The model under review builds one solid part; all positions refer to its coordinate system, in mm. A direction names the side the tool comes from. Round coordinates to 2 decimals unless told otherwise and drop trailing zeros. Loops run counter-clockwise (first coordinate to the right, second up) from the corner with the lowest first, then second, coordinate; pieces in that order, holes last. Notation, with made-up numbers: M 8.25,16.25 L 67.25,16.25 A14 cw 67.25,21.25 Z; hole C 67,62.5 d1. An arc over 180 degrees is marked long. Return JSON: item names as keys, results as strings. Group by question number.
Q1. To check wall thickness, follow line 1 along X through (y, z) = (16.3, 0); line 2 along Y through (x, z) = (17.5, 47); line 3 along Y through (x, z) = (25, 32.25). State the ranges of each line that lie inside material, in increasing order.
Q2. Consider section C-C (y = -46). State the section outline as (x, z) points.
Q3. Consider section B-B (z = -33). Count the separate pieces of the cut face and the enclosed holes in it, and give its area (3 significant figures).
Q4. Draft analysis for pull direction Y (two halves, no side actions). For faces 1 (the face through (15.69, -17.46, -49.84)), 2 (the face through (-34, -86.15, -14)), 3 (the face through (27.147, 68.608, 32.475)), state which applies: pulls with the +Y half, pulls with the -Y half, needs draft (parallel to the pull), parting line crosses it, or undercut.
Q5. Clearance check with flat-ended pins moving along their axes: pin 1 Ø5.5 at (x, y) = (25, 86.5) entering from -Z; pin 2 Ø4 at (x, y) = (25, 68.5) entering from +Z; pin 3 Ø1 at (x, y) = (1.5, 49.5) entering from +Z; pin 4 Ø5 at (x, y) = (5.5, 30) entering from +Z. State where each tip first meets the part, or that it passes through.
Q6. Consider section A-A (y = 68.5). State the section outline as (x, z) points, and give its area (3 significant figures).
Q7. For faces 4 (the face through (29.23, -0.21, -31.88)), 5 (the face through (-35, -92.5, 16)), 6 (the face through (-34, 13.85, -14)), 7 (the face through (-23, -62.5, 37)), list the 3-axis set-ups (+Z, -Z, +X, -X, +Y, -Y) from which the entire face can be reached by the end or side of a thin tool; tool diameter is ignored.
from build123d import *

# Parameters (mm, degrees)
SKETCH1_R                      = 45.25
SKETCH1_R_2                    = 38.25
BOSS_EXTRUDE1_DEPTH            = 92.5
BOSS_EXTRUDE2_START            = -6.35
SKETCH2_R                      = 38.25
SKETCH2_R_2                    = 36.25
BOSS_EXTRUDE2_DEPTH            = 100
CUT_EXTRUDE3_START             = -44
SKETCH6_R                      = 39.25
SKETCH6_R_2                    = 38.25
CUT_EXTRUDE3_DEPTH             = 44
SKETCH7_R                      = 17.5
CUT_EXTRUDE4_DEPTH             = 113.478331247
SKETCH8_R                      = 45.25
SKETCH8_R_2                    = 43.25
CUT_EXTRUDE5_DEPTH             = 30
SKETCH9_R                      = 45.25
SKETCH9_R_2                    = 43.25
CUT_EXTRUDE6_DEPTH             = 15
SKETCH10_R                     = 52.25
SKETCH10_R_2                   = 43.25
SKETCH10_R_3                   = 1.75
BOSS_EXTRUDE3_DEPTH            = 5
CBORE_FOR_M4_SHCS1_D           = 4.3
CBORE_FOR_M4_SHCS1_DEPTH       = 100.101198794
CBORE_FOR_M4_SHCS1_CBORE_D     = 8
CBORE_FOR_M4_SHCS1_CBORE_DEPTH = 4
CBORE_FOR_M4_SHCS1_TIP         = 1.291850331


with BuildPart() as part:
    # Sketch1 → Boss-Extrude1 (new, symmetric)
    with BuildSketch(Plane(origin=(0, 0, 0), x_dir=(1, 0, 0), z_dir=(0, 1, 0))):
        with Locations(Location((0, 0, 0), (0, 0, 270))):
            Circle(SKETCH1_R)
        with Locations(Location((0, 0, 0), (0, 0, 270))):
            Circle(SKETCH1_R_2, mode=Mode.SUBTRACT)
    extrude(amount=BOSS_EXTRUDE1_DEPTH, both=True)

    # Sketch2 → Boss-Extrude2 (add)
    with BuildSketch(Plane.XZ.offset(92.5).offset(BOSS_EXTRUDE2_START)):
        with Locations(Location((0, 0, 0), (0, 0, 270))):
            Circle(SKETCH2_R)
        with Locations(Location((0, 0, 0), (0, 0, 270))):
            Circle(SKETCH2_R_2, mode=Mode.SUBTRACT)
    extrude(amount=-BOSS_EXTRUDE2_DEPTH)

    # Sketch6 → Cut-Extrude3 (cut)
    with BuildSketch(Plane(origin=(0, 92.5, 0), x_dir=(1, 0, 0), z_dir=(0, 1, 0)).offset(CUT_EXTRUDE3_START)):
        with Locations(Location((0, 0, 0), (0, 0, 270))):
            Circle(SKETCH6_R)
        with Locations(Location((0, 0, 0), (0, 0, 90))):
            Circle(SKETCH6_R_2, mode=Mode.SUBTRACT)
    extrude(amount=CUT_EXTRUDE3_DEPTH, mode=Mode.SUBTRACT)

    # Sketch7 → Cut-Extrude4 (cut, through all)
    with BuildSketch(Plane(origin=(0, 0, 0), x_dir=(0, 0, -1), z_dir=(1, 0, 0))):
        with Locations(Location((0, 38.75, 0), (0, 0, 33.858436659))):
            Circle(SKETCH7_R)
    extrude(amount=-CUT_EXTRUDE4_DEPTH, mode=Mode.SUBTRACT)

    # Sketch8 → Cut-Extrude5 (cut)
    with BuildSketch(Plane(origin=(0, 92.5, 0), x_dir=(1, 0, 0), z_dir=(0, 1, 0))):
        with Locations(Location((0, 0, 0), (0, 0, 270))):
            Circle(SKETCH8_R)
        with Locations(Location((0, 0, 0), (0, 0, 270))):
            Circle(SKETCH8_R_2, mode=Mode.SUBTRACT)
    cut_extrude5 = extrude(amount=-CUT_EXTRUDE5_DEPTH, mode=Mode.SUBTRACT)

    # Mirror1: Cut-Extrude5 across plane
    add(cut_extrude5.mirror(Plane.ZX), mode=Mode.SUBTRACT)

    # Sketch9 → Cut-Extrude6 (cut, symmetric)
    with BuildSketch(Plane(origin=(0, 0, 0), x_dir=(1, 0, 0), z_dir=(0, 1, 0))):
        with Locations(Location((0, 0, 0), (0, 0, 270))):
            Circle(SKETCH9_R)
        with Locations(Location((0, 0, 0), (0, 0, 270))):
            Circle(SKETCH9_R_2, mode=Mode.SUBTRACT)
    extrude(amount=CUT_EXTRUDE6_DEPTH, both=True, mode=Mode.SUBTRACT)

    # Sketch10 → Boss-Extrude3 (add)
    with BuildSketch(Plane(origin=(0, 15, 0), x_dir=(-1, 0, 0), z_dir=(0, -1, 0))):
        with Locations(Location((0, 0, 0), (0, 0, 90))):
            Circle(SKETCH10_R)
        with Locations(Location((0, 0, 0), (0, 0, 270))):
            Circle(SKETCH10_R_2, mode=Mode.SUBTRACT)
        with Locations(Location((-48.75, 0, 0), (0, 0, 90))):
            Circle(SKETCH10_R_3, mode=Mode.SUBTRACT)
    boss_extrude3 = extrude(amount=-BOSS_EXTRUDE3_DEPTH)

    # Mirror2: Boss-Extrude3 across plane
    add(boss_extrude3.mirror(Plane.ZX))

    # CBORE for M4 SHCS1
    with Locations(Plane(origin=(401.677021233, -407.224238547, 50.050599397), x_dir=(0.16757219303491572, 0.985859807539322, 0), z_dir=(0, 0, 1))):
        with Locations((405.876811742, 451.068889591), (423.622288278, 454.085189065)):
            CounterBoreHole(CBORE_FOR_M4_SHCS1_D / 2, CBORE_FOR_M4_SHCS1_CBORE_D / 2, CBORE_FOR_M4_SHCS1_CBORE_DEPTH, depth=CBORE_FOR_M4_SHCS1_DEPTH)
            with Locations((0, 0, -(CBORE_FOR_M4_SHCS1_DEPTH + CBORE_FOR_M4_SHCS1_TIP / 2))):  # 118° drill point
                Cone(0, CBORE_FOR_M4_SHCS1_D / 2, CBORE_FOR_M4_SHCS1_TIP, mode=Mode.SUBTRACT)


solid = part.part
Values:
{
 "1": {"line 1": "x = -52.25 to -38.25, 38.25 to 47, 50.5 to 52.25", "line 2": "y = -20 to -15, 15 to 20", "line 3": "y = -92.5 to 66.35, 70.65 to 84.35, 88.65 to 92.5"},
 "2": {"outline": "C 0,0 d90.5; hole C 0,0 d72.5"},
 "3": {"separate pieces": "2", "enclosed holes": "2", "area": "4,620 mm2"},
 "4": {"face 1": "needs draft", "face 2": "pulls with the -Y half", "face 3": "undercut"},
 "5": {"pin 1": "stops at z = -37.09", "pin 2": "passes through", "pin 3": "stops at z = 45.24", "pin 4": "stops at z = 45.15"},
 "6": {"outline": "M 22.85,-36.72 L 22.85,-31.91 A39.25 cw long 22.85,31.91 L 22.85,36.72 A43.25 ccw long Z; M 27.15,-33.67 A43.25 ccw 27.15,33.67 L 27.15,28.35 A39.25 cw 27.15,-28.35 Z", "area": "993 mm2"},
 "7": {"face 4": "none", "face 5": "+Z, -Z, +X, -X, -Y", "face 6": "+Y", "face 7": "-Y"}
}
